Geometry check sheet. Reference: the model listing, model coordinates, mm. A direction names the side the tool comes from. Round coordinates to 2 decimals unless told otherwise and drop trailing zeros. Order: outer loops, then holes, each group sorted by start corner. A loop starts at its lowest first (then second) coordinate and runs counter-clockwise, first axis right, second up. Notation, with made-up numbers: (-28, -14.5) - (3, -14.5) arc R20 cw to (3, 8.5) - close; hole circle Ø1 at (4, -40). An arc over 180 degrees is marked (long way). Return JSON: item names as keys, results as strings. Group by question number.
Q1. Material ranges on line 1 along Z through (x, y) = (79, -177.5); line 2 along X through (y, z) = (-27, 31.5); line 3 along Z through (x, y) = (-29, -149), recorded low to high.
Q2. Sectioned sample at C-C, the plane z = 112. Record the cut outline in (x, y).
Q3. Gauge pin test, flat ends, axial feed: pin 1 Ø4 at (x, z) = (31.5, 105.5) entering from -Y; pin 2 Ø16.5 at (x, y) = (58, -103) entering from +Z; pin 3 Ø0.5 at (x, y) = (-16.5, 0) entering from -Z. Record the tip position at first contact, or that the pin passes through.
Q4. Sectioned sample at A-A, the plane x = -8. Record the cut outline in (y, z), then the cut area to 3 significant figures.
Q5. Draft check along Z on faces 1 (the flat face through (-18, 0.499, 124)), 2 (the flat face through (77, -157, 59.663)), 3 (the flat face through (-18, -176, 96.22)). Enter one of: pulls with the +Z half, pulls with the -Z half, needs draft (parallel to the pull), parting line crosses it, or undercut.
Q6. Sectioned sample at B-B, the plane y = -199.5. Record the cut outline in (x, z), then the cut area to 3 significant figures.
Q7. Sectioned sample at D-D, the plane x = 68.5. Record the cut outline in (y, z).
Q8. Tool access check on faces 4 (the flat face through (66.1, -108.32, 78.2)), 5 (the flat face through (-43, -111, 59.663)), 6 (the flat face through (-0.03, -195, 86)), 7 (the flat face through (92.941, -108, 29)), 8 (the flat face through (47, -108, 0)). Record the directions out of +Z, -Z, +X, -X, +Y, -Y that give a thin tool (end or side, any length) a straight path to the whole face; none if there is none.
```python
from build123d import *

# Parameters (mm, degrees)
F0_W      = 92.9407775402
F0_H      = 151.2379273772
F1_DEPTH  = 219.7186052799
F3_DEPTH  = 55.0180487335
F4_DEPTH  = 86.1361920834
F6_DEPTH  = 36.5569889545
F8_DEPTH  = 101.3751477003
F9_W      = 86.8442915817
F9_H      = 59.6628896892
F10_DEPTH = 283.972
F12_DEPTH = 86.106
F14_DEPTH = 220.218


with BuildPart() as f1:
    # F0 (on Front) → F1 (new body)
    with BuildSketch(Plane.XZ):
        with Locations((46.4703887701, 75.6189636886)):
            Rectangle(F0_W, F0_H)
    extrude(amount=F1_DEPTH)

    # F2 (on face) → F3 (cut)
    with BuildSketch(Plane.XY.offset(151.2379273772)):
        Polygon((92.9407775402, -219.7186052799), (92.9407775402, 0), (0, -219.7186052799), align=None)
    extrude(amount=-F3_DEPTH, mode=Mode.SUBTRACT)

    # F4 (add): a face of the model
    f4_faces = [f1.faces().sort_by_distance(p)[0] for p in [
        (0, -109.85930264, 75.6189636886),
    ]]
    extrude(f4_faces, amount=F4_DEPTH)

    # F5 (on face) → F6 (cut)
    with BuildSketch(Plane.XY.offset(96.2198786438)):
        Polygon((158.591479063, 33.0015420914), (92.9407775402, 0), (31.3818752766, -248.4212368727), (158.591479063, -248.4212368727), align=None)
        Polygon((158.591479063, 33.0015420914), (92.9407775402, 0), (92.9407775402, -219.7186052799), (38.4944012231, -219.7186052799), (31.3818752766, -248.4212368727), (158.591479063, -248.4212368727), align=None)
    extrude(amount=-F6_DEPTH, mode=Mode.SUBTRACT)

    # F7 (on face) → F8 (cut)
    with BuildSketch(Plane(origin=(-86.1361920834, 0, 0), x_dir=(0, -1, 0), z_dir=(-1, 0, 0))):
        Polygon((29.3830856681, 269.2216336727), (0, 151.2379273772), (219.7186052799, 151.2379273772), (219.7186052799, 65.060840155), (247.8701323271, 54.019369185), (303.3900067808, 195.5738098548), align=None)
    extrude(amount=-F8_DEPTH, mode=Mode.SUBTRACT)

    # F9 (on face) → F10 (cut)
    with BuildSketch(Plane.XZ.offset(219.7186052799)):
        with Locations((-42.7140462925, 29.8314448446)):
            Rectangle(F9_W, F9_H)
    extrude(amount=-F10_DEPTH, mode=Mode.SUBTRACT)

    # F11 (on face) → F12 (cut)
    with BuildSketch(Plane(origin=(-86.1361920834, 0, 0), x_dir=(0, -1, 0), z_dir=(-1, 0, 0))):
        Polygon((219.7186052799, 151.2379273772), (0, 151.2379273772), (219.7186052799, 59.6628896892), align=None)
    extrude(amount=-F12_DEPTH, mode=Mode.SUBTRACT)

    # F13 (on face) → F14 (join)
    with BuildSketch(Plane.XZ.offset(219.7186052799)):
        Polygon((-35.4988574982, 96.2198786438), (-0.0301920834, 96.2198786438), (-0.0301920834, 151.2379273772), (0, 151.2379273772), (0, 151.3858735561), (-35.4988574982, 151.3858735561), align=None)
    extrude(amount=-F14_DEPTH)


solid = f1.part
```
Reply:
{
 "1": {"line 1": "0 to 59.66", "line 2": "0.71 to 92.94", "line 3": "59.66 to 89.14, 96.22 to 151.39"},
 "2": {"outline": "(-86.14, -94.14) - (-35.5, -94.14) - (-35.5, -219.72) - (0, -219.72) - (92.94, 0) - (-0.03, 0) - (-0.03, 0.5) - (-35.5, 0.5) - (-35.5, 0) - (-86.14, 0) - close"},
 "3": {"pin 1": "y = -149.98", "pin 2": "z = 151.24", "pin 3": "z = 59.66"},
 "4": {"outline": "(-219.72, 59.66) - (0, 59.66) - (0, 96.22) - (0.5, 96.22) - (0.5, 151.39) - (-219.72, 151.39) - (-219.72, 96.22) - (-132.01, 96.22) - close", "area": "18,600 mm^2"},
 "5": {"face 1": "needs draft", "face 2": "pulls with the +Z half", "face 3": "undercut"},
 "6": {"outline": "(-86.14, 59.66) - (0.71, 59.66) - (0.71, 0) - (92.94, 0) - (92.94, 59.66) - (43.5, 59.66) - (43.5, 96.22) - (8.55, 96.22) - (8.55, 151.24) - (0, 151.24) - (0, 151.39) - (-35.5, 151.39) - (-35.5, 96.22) - (-0.03, 96.22) - (-0.03, 68.09) - (-86.14, 68.09) - close", "area": "10,200 mm^2"},
 "7": {"outline": "(-219.72, 0) - (0, 0) - (0, 151.24) - (-57.78, 151.24) - (-57.78, 96.22) - (-98.63, 96.22) - (-98.63, 59.66) - (-219.72, 59.66) - close"},
 "8": {"face 4": "+Z, +X, -Y", "face 5": "-Z, -X, +Y, -Y", "face 6": "-X, -Y", "face 7": "+Z, -Z, +X, +Y, -Y", "face 8": "-Z, +X, -X, +Y, -Y"}
}
